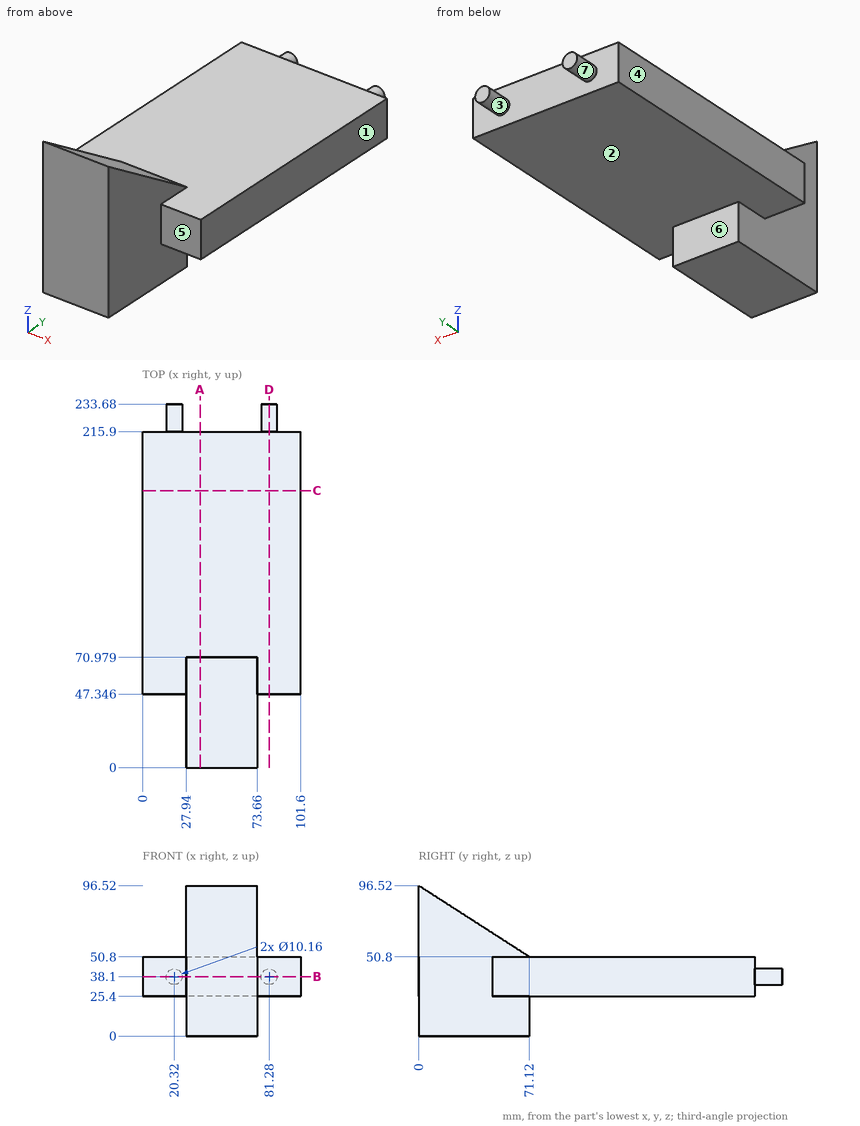
Here's the drawing with two shaded views (mm, measured from the low corner). I have some questions. A direction names the side the tool comes from. Coordinates: 2 decimals unless noted, no trailing zeros. Order: outer loops, then holes, each group sorted by start corner. A loop starts at its lowest first (then second) coordinate and runs counter-clockwise, first axis right, second up.
Q1. Suppose I cut it at D-D on x = 81.28. Please give me the cut outline in (y, z), and give its area (3 significant figures).
Q2. Suppose I cut it at A-A on x = 37. Please give me the cut outline in (y, z), and give its area (3 significant figures).
Q3. Please list where these lines run through material, in increasing order: L1, parallel to Z at x = 34, y = 178.5; L2, parallel to X at y = 29.5, z = 6.5; L3, parallel to Y at x = 59, z = 17.
Q4. Will these pins go through, and if not, where does the flat tip stop? pin 1 (21.5 mm diameter, centred on y = 20, z = 30.5, fed in from -X); pin 2 (1 mm diameter, centred on y = 35.5, z = 69, fed in from +X); pin 3 (4 mm diameter, centred on x = 57.5, y = 201.5, fed in from -Z).
Q5. Suppose I cut it at C-C on y = 178. Please give me the cut outline in (x, z), and give its area (3 significant figures).
Q6. Which directions (+Z, -Z, +X, -X, +Y, -Y) give clear straight access to the entire face, cutting with the end or side of a thin tool? Please do the marked faces 4, 5, 6 and 7.
Q7. Suppose I cut it at B-B on z = 38.1. Please give me the cut outline in (x, y).
Q8. Thinking about a two-plate mould opening in X: for the marked faces 1, 2 and 3, which applies, released by +X, released by -X, zero draft, split by the parting line, or undercut?
Answer:
1. outline: (47.35, 25.4) - (215.9, 25.4) - (215.9, 33.02) - (233.68, 33.02) - (233.68, 43.18) - (215.9, 43.18) - (215.9, 50.8) - (47.35, 50.8) - close
1. area: 4,460 mm2
2. outline: (0, 0) - (70.98, 0) - (70.98, 25.4) - (215.9, 25.4) - (215.9, 50.8) - (71.12, 50.8) - (0, 96.52) - close
2. area: 8,910 mm2
3. L1: z = 25.4 to 50.8
3. L2: x = 27.94 to 73.66
3. L3: y = 0 to 70.98
4. pin 1: stops at x = 27.94
4. pin 2: stops at x = 73.66
4. pin 3: stops at z = 25.4
5. outline: (0, 25.4) - (101.6, 25.4) - (101.6, 50.8) - (0, 50.8) - close
5. area: 2,580 mm2
6. face 4: +Z, -Z, -X, +Y, -Y
6. face 5: +Z, -Z, +X, -Y
6. face 6: -Z, +X, -X, +Y
6. face 7: +Y
7. outline: (0, 47.35) - (27.94, 47.35) - (27.94, 0) - (73.66, 0) - (73.66, 47.35) - (101.6, 47.35) - (101.6, 215.9) - (86.36, 215.9) - (86.36, 233.68) - (76.2, 233.68) - (76.2, 215.9) - (25.4, 215.9) - (25.4, 233.68) - (15.24, 233.68) - (15.24, 215.9) - (0, 215.9) - close
8. face 1: released by +X
8. face 2: zero draft
8. face 3: undercut
